Part model, mm, in its own coordinate system. A direction names the side the tool comes from. Give positions to 0.01 mm unless a question says otherwise; leave off trailing zeros. Order: outer loops, then holes, each group sorted by start corner. A loop starts at its lowest first (then second) coordinate and runs counter-clockwise, first axis right, second up. Notation, with made-up numbers: (21, 36.25) - (29, 36.25) arc R28 ccw to (29, 56.25) - close; hole circle Ø2 at (65, 69). An arc over 180 degrees is marked (long way). Use one line per item in the form item = value. Start each with the question number.
1. Drill centre lines: line 1 (X direction, y = 43, z = 0); line 2 (Z direction, x = -54, y = 42.5); line 3 (Z direction, x = -0.5, y = 42). Where is each one in solid material? Low to high.
2. Tool access for faces 1 (the face through (-44, 27, 7.469)), 2 (the face through (-42, 27, -17.031)), 3 (the face through (-43, 27, 16.969)), 4 (the face through (20.795, 27, 50)): list every direction of +Z, -Z, +X, -X, +Y, -Y with a clear straight run to the whole face (end or side of a thin tool).
3. Band-saw the part on D-D, the plane z = 0. List the corners of the cut face in (x, y).
4. Band-saw the part on A-A, the plane x = 0. List the corners of the cut face in (y, z), plus the area to 3 significant figures.
5. Band-saw the part on C-C, the plane y = 19.5. List the corners of the cut face in (x, z).
6. Band-saw the part on B-B, the plane z = 41. List the corners of the cut face in (x, y).
7. Pull direction Z, two halves, no side cores. Call faces 5 (the face through (23.76, 27.12, -25.7)), 6 (the face through (-19.524, 27.115, -4.336)), 7 (the face through (-14.05, 4.51, 67.72)), 8 (the face through (-45, 27, -7.531)): +Z half, -Z half, draft (parallel to the pull), parting line (faces both ways), or undercut.
8. Pin check, flat tips, straight feed: P1, Ø5, axis at x = 8, y = 5.5, coming from the +Z side; P2, Ø4, axis at x = 5.5, y = 46, coming from the -Z side; P3, Ø1.5, axis at y = 17.5, z = -15, coming from the -X side. Stop position of each tip, or through.
from build123d import *

# Parameters (mm, degrees)
SKETCH2_R           = 20
BOSS_EXTRUDE3_DEPTH = 55
FILLET1_R           = 15


with BuildPart() as part:
    # Sketch2 → Boss-Extrude3 (new body)
    with BuildSketch(Plane(origin=(0, 0, 0), x_dir=(1, 0, 0), z_dir=(0, 1, 0))):
        with BuildLine():
            Line((-20.795375831, -28.152306194), (-20.795375831, -72))
            Line((-20.795375831, -72), (-7.5, -72))
            Line((-7.5, -72), (-7.5, -34.186985828))
            ThreePointArc((-7.5, -34.186985828), (0, -35), (7.5, -34.186985828))
            Line((7.5, -34.186985828), (7.5, -72))
            Line((7.5, -72), (20.795375831, -72))
            Line((20.795375831, -72), (20.795375831, -28.152306194))
            ThreePointArc((20.795375831, -28.152306194), (23.114885766, 26.281211083), (-30.576990341, 17.030785705))
            Line((-30.576990341, 17.030785705), (-54.576990341, 17.030785705))
            ThreePointArc((-54.576990341, 17.030785705), (-72.004836058, 0.048305486), (-54.611203279, -16.969214295))
            Line((-54.611203279, -16.969214295), (-30.611203279, -16.969214295))
            ThreePointArc((-30.611203279, -16.969214295), (-26.304457418, -23.088428269), (-20.795375831, -28.152306194))
        make_face()
        with BuildLine():
            ThreePointArc((-34.180128859, 7.531187899), (-34.999985436, 0.031929592), (-34.193812975, -7.468812101))
            Line((-34.193812975, -7.468812101), (-54.999991154, -7.468812101))
            ThreePointArc((-54.999991154, -7.468812101), (-62.499994275, 0.038036202), (-54.986307038, 7.531187899))
            Line((-54.986307038, 7.531187899), (-34.180128859, 7.531187899))
        make_face(mode=Mode.SUBTRACT)
        with Locations(Location((0, 0, 0), (0, 0, 270))):
            Circle(SKETCH2_R, mode=Mode.SUBTRACT)
    extrude(amount=BOSS_EXTRUDE3_DEPTH)

    # Fillet1
    fillet1_edges = [part.edges().sort_by_distance(p)[0] for p in [
        (-14.147687915, 0, 72),
        (14.147687915, 0, 72),
        (14.147687915, 55, 72),
        (-14.147687915, 55, 72),
    ]]
    fillet(fillet1_edges, radius=FILLET1_R)


solid = part.part
From the geometry:
q1.line_1 = -72 to -62.5, -35 to -20, 20 to 35
q1.line_2 = -17.03 to -7.53, 7.47 to 16.97
q1.line_3 = -35 to -19.99, 19.99 to 35
q2.face_1 = +Y, -Y
q2.face_2 = -Z, -X, +Y, -Y
q2.face_3 = +Z, -X, +Y, -Y
q2.face_4 = +Z, +X, +Y, -Y
q3.outline = (-72, 0) - (-62.5, 0) - (-62.5, 55) - (-72, 55) - close; (-35, 0) - (-20, 0) - (-20, 55) - (-35, 55) - close; (20, 0) - (35, 0) - (35, 55) - (20, 55) - close
q4.outline = (0, -35) - (55, -35) - (55, -20) - (0, -20) - close; (0, 20) - (55, 20) - (55, 35) - (0, 35) - close
q4.area = 1,650 mm²
q5.outline = (-54.61, 16.97) arc R17 ccw (long way) to (-54.58, -17.03) - (-30.58, -17.03) arc R35 ccw (long way) to (20.8, 28.15) - (20.8, 72) - (7.5, 72) - (7.5, 34.19) arc R35 ccw to (-7.5, 34.19) - (-7.5, 72) - (-20.8, 72) - (-20.8, 28.15) arc R35 ccw to (-30.61, 16.97) - close; hole (-55, 7.47) arc R7.5 ccw to (-54.99, -7.53) - (-34.18, -7.53) arc R35 cw to (-34.19, 7.47) - close; hole circle Ø40 at (0, 0)
q6.outline = (-20.8, 0) - (-7.5, 0) - (-7.5, 55) - (-20.8, 55) - close; (7.5, 0) - (20.8, 0) - (20.8, 55) - (7.5, 55) - close
q7.face_5 = parting line
q7.face_6 = undercut
q7.face_7 = +Z half
q7.face_8 = undercut
q8.P1 = 70.27
q8.P2 = -34.82
q8.P3 = -64.33
